```python
from build123d import *

# Parameters (mm, degrees)
SKETCH_W     = 14.6
SKETCH_H     = 8.6
SKETCH_R     = 3.2
PAD_DEPTH    = 2.6
SKETCH001_W  = 8.6
SKETCH001_H  = 8.6
SKETCH001_R  = 3.2
PAD001_DEPTH = 4.4


with BuildPart() as part:
    # Sketch → Pad (new body)
    with BuildSketch(Plane.XY):
        Rectangle(SKETCH_W, SKETCH_H)
        Circle(SKETCH_R, mode=Mode.SUBTRACT)
    extrude(amount=PAD_DEPTH)

    # Sketch001 (on Face7 of Pad) → Pad001 (join)
    with BuildSketch(Plane.XY.offset(2.6)):
        Rectangle(SKETCH001_W, SKETCH001_H)
        Circle(SKETCH001_R, mode=Mode.SUBTRACT)
    extrude(amount=PAD001_DEPTH)


solid = part.part
```
Here's how the part is built. I have some questions about the finished solid (model axes, mm). A direction names the side the tool comes from. Coordinates: 2 decimals unless noted, no trailing zeros. Write each loop counter-clockwise with the first axis right and the second up, starting at its lowest first coordinate (ties: lowest second). Pieces come first, ordered by that corner, then holes. Notation, with made-up numbers: (36, 69) -> (66, 69) arc R23 cw to (66, 107) -> close; hole circle Ø3 at (76.5, 45). An arc over 180 degrees is marked (long way). Use a Markdown table: item, result. Add a question column.
(1) For faces 4 (the flat face through (6, 0, 2.6)), 5 (the flat face through (-6, 0, 2.6)), 6 (the flat face through (-3.35, 0.06, 0)), which set-ups out of +Z, -Z, +X, -X, +Y, -Y let a thin tool reach every point of the face, with its end or its side?
(2) If we section it at B-B, the plane x = 0: Write out the boundary of the cut face in (y, z).
(3) We'd pull the mould along X, two halves only. Please class faces 1 (the flat face through (0, -4.3, 3)), 2 (the cylindrical face through (-2.539, -1.947, 3.451)), 3 (the flat face through (-4.3, 0, 5)): +X half, -X half, draft (parallel to the pull), parting line (faces both ways), or undercut.
(4) If we section it at D-D, the plane y = -3.5: Write out the boundary of the cut face in (x, z), and give its area (3 significant figures).
(5) I'm going to push flat-ended pins straight in: P1, Ø2, axis at y = 0.5, z = 4, coming from the -X side; P2, Ø2, axis at y = -0.5, z = 5, coming from the +X side. Where does each tip first touch, or does it pass through?
(6) If we section it at A-A, the plane y = 0: Write out the boundary of the cut face in (x, z).
(7) Please list where these lines run through material, in increasing order: line 1 (Y direction, x = 0, z = 1.75); line 2 (X direction, y = 1.5, z = 4); line 3 (Z direction, x = -6.5, y = 0).
(8) If we section it at C-C, the plane z = 3.25: Write out the boundary of the cut face in (x, y), and give its area (3 significant figures).
Outcome:
| question | item | result |
|---|---|---|
| 1 | face 4 | +Z, +X, +Y, -Y |
| 1 | face 5 | +Z, -X, +Y, -Y |
| 1 | face 6 | -Z, +X, -X, +Y, -Y |
| 2 | outline | (-4.3, 0) -> (-3.2, 0) -> (-3.2, 7) -> (-4.3, 7) -> close; (3.2, 0) -> (4.3, 0) -> (4.3, 7) -> (3.2, 7) -> close |
| 3 | face 1 | draft |
| 3 | face 2 | undercut |
| 3 | face 3 | -X half |
| 4 | outline | (-7.3, 0) -> (7.3, 0) -> (7.3, 2.6) -> (4.3, 2.6) -> (4.3, 7) -> (-4.3, 7) -> (-4.3, 2.6) -> (-7.3, 2.6) -> close |
| 4 | area | 75.8 mm^2 |
| 5 | P1 | stops at x = -4.3 |
| 5 | P2 | stops at x = 4.3 |
| 6 | outline | (-7.3, 0) -> (-3.2, 0) -> (-3.2, 7) -> (-4.3, 7) -> (-4.3, 2.6) -> (-7.3, 2.6) -> close; (3.2, 0) -> (7.3, 0) -> (7.3, 2.6) -> (4.3, 2.6) -> (4.3, 7) -> (3.2, 7) -> close |
| 7 | line 1 | y = -4.3 to -3.2, 3.2 to 4.3 |
| 7 | line 2 | x = -4.3 to -2.83, 2.83 to 4.3 |
| 7 | line 3 | z = 0 to 2.6 |
| 8 | outline | (-4.3, -4.3) -> (4.3, -4.3) -> (4.3, 4.3) -> (-4.3, 4.3) -> close; hole circle Ø6.4 at (0, 0) |
| 8 | area | 41.8 mm^2 |
